from build123d import *

# Parameters (mm, degrees)
F1_DEPTH = 101.6
F2_R     = 25.4
F3_DEPTH = 76.201
F4_W     = 25.4
F4_H     = 50.8
F5_DEPTH = 177.801


with BuildPart() as f1:
    # F0 (on Top) → F1 (new body)
    with BuildSketch(Plane.XY):
        Polygon((0, 25.4), (0, 0), (152.4, 0), (152.4, 76.2), (-25.4, 76.2), (-25.4, 25.4), align=None)
    extrude(amount=F1_DEPTH)

    # F2 (on face) → F3 (cut, through all)
    with BuildSketch(Plane.XZ):
        with BuildLine():
            Line((25.4, 50.8), (25.4, 0))
            Line((25.4, 0), (50.8, 0))
            Line((50.8, 0), (50.8, 50.8))
            ThreePointArc((50.8, 50.8), (38.1, 63.5), (25.4, 50.8))
        make_face()
        with Locations((101.6, 50.8)):
            Circle(F2_R)
    extrude(amount=-F3_DEPTH, mode=Mode.SUBTRACT)

    # F4 (on face) → F5 (cut, through all)
    with BuildSketch(Plane.YZ.offset(152.4)):
        with Locations((63.5, 50.8)):
            Rectangle(F4_W, F4_H)
    extrude(amount=-F5_DEPTH, mode=Mode.SUBTRACT)


solid = f1.part
Could you check a few things on this model? Use its own coordinates, in mm. A direction names the side the tool comes from. Round coordinates to 2 decimals unless told otherwise and drop trailing zeros. Write each loop counter-clockwise with the first axis right and the second up, starting at its lowest first coordinate (ties: lowest second). Pieces come first, ordered by that corner, then holes. Notation, with made-up numbers: (20, -24) - (40, -24) arc R26 ccw to (40, 6) - close; hole circle Ø3 at (0, 56). An arc over 180 degrees is marked (long way). Put each result on its own line as item: value. Start each with the question number.
(1) For faces 1 (the flat face through (102, 63, 25.4)), 2 (the flat face through (50.8, 29, 25)), 3 (the flat face through (0, 13, 50)), which set-ups out of +Z, -Z, +X, -X, +Y, -Y let a thin tool reach every point of the face, with its end or its side?
(2) Thinking about a two-plate mould opening in Z: for faces 4 (the flat face through (62, 39, 101.6)), 5 (the flat face through (65, 76.2, 89)), 6 (the flat face through (139, 50.8, 50)), which applies, released by +Z, released by -Z, zero draft, split by the parting line, or undercut?
(3) I want a section at D-D, the plane x = 125. Please give me the cut outline in (y, z), plus the area to 3 significant figures.
(4) I need wall thicknesses on probe 1 along X at (y, z) = (31, 50.8); probe 2 along X at (y, z) = (10, 50); probe 3 along X at (y, z) = (14, 5). Which ranges of each line are inside material? Lowest first, please.
(5) I want a section at B-B, the plane z = 71. Please give me the cut outline in (x, y), plus the area to 3 significant figures.
(6) I want a section at C-C, the plane x = -5.5. Please give me the cut outline in (y, z).
(7) I want a section at A-A, the plane y = 44. Please give me the cut outline in (x, z), plus the area to 3 significant figures.
(8) Will these pins go through, and if not, where does the flat tip stop? pin 1 (12.5 mm diameter, centred on y = 16.5, z = 75.5, fed in from -X); pin 2 (15 mm diameter, centred on x = 137, z = 56.5, fed in from +Y); pin 3 (12.5 mm diameter, centred on x = -13.5, z = 61.5, fed in from -Y).
Here are the results:
1. face 1: +X, -X, +Y
1. face 2: -Z, +Y, -Y
1. face 3: +Z, -Z, -X, -Y
2. face 4: released by +Z
2. face 5: zero draft
2. face 6: undercut
3. outline: (0, 0) - (76.2, 0) - (76.2, 25.4) - (50.8, 25.4) - (50.8, 40.92) - (0, 40.92) - close; (0, 60.68) - (50.8, 60.68) - (50.8, 76.2) - (76.2, 76.2) - (76.2, 101.6) - (0, 101.6) - close
3. area: 5,450 mm^2
4. probe 1: x = -25.4 to 25.4, 50.8 to 76.2, 127 to 152.4
4. probe 2: x = 0 to 25.4, 50.8 to 76.21, 126.99 to 152.4
4. probe 3: x = 0 to 25.4, 50.8 to 152.4
5. outline: (-25.4, 25.4) - (0, 25.4) - (0, 0) - (86.2, 0) - (86.2, 50.8) - (-25.4, 50.8) - close; (117, 0) - (152.4, 0) - (152.4, 50.8) - (117, 50.8) - close
5. area: 6,820 mm^2
6. outline: (25.4, 0) - (76.2, 0) - (76.2, 25.4) - (50.8, 25.4) - (50.8, 76.2) - (76.2, 76.2) - (76.2, 101.6) - (25.4, 101.6) - close
7. outline: (-25.4, 0) - (25.4, 0) - (25.4, 50.8) arc R12.7 cw to (50.8, 50.8) - (50.8, 0) - (152.4, 0) - (152.4, 101.6) - (-25.4, 101.6) - close; hole circle Ø50.8 at (101.6, 50.8)
7. area: 14,500 mm^2
8. pin 1: stops at x = 0
8. pin 2: stops at y = 50.8
8. pin 3: stops at y = 25.4
